```python
from build123d import *
from build123d.topology import SkipClean

# Parameters (mm, degrees)
CROQUIS2_R              = 11.9
SALIENTE_EXTRUIR1_DEPTH = 30
CROQUIS3_R              = 3
SALIENTE_EXTRUIR2_DEPTH = 1.5
CROQUIS4_R              = 1
CORTAR_EXTRUIR1_DEPTH   = 36.713722853
CROQUIS5_R              = 1.2
CORTAR_EXTRUIR2_DEPTH   = 5
CROQUIS7_R              = 4.5
SALIENTE_EXTRUIR3_DEPTH = 1.7
CORTAR_EXTRUIR3_REACH   = 39.222
CROQUIS8_R              = 1
SALIENTE_EXTRUIR4_DEPTH = 5
CORTAR_EXTRUIR4_REACH   = 41.632
CROQUIS10_R             = 0.5
CORTAR_EXTRUIR5_DEPTH   = 3
CORTAR_EXTRUIR7_DEPTH   = 2
SALIENTE_EXTRUIR5_START = 1
SALIENTE_EXTRUIR5_DEPTH = 1
CROQUIS16_R             = 1
SALIENTE_EXTRUIR8_DEPTH = 0.4
CROQUIS17_R             = 1
SALIENTE_EXTRUIR9_DEPTH = 45
REDONDEO4_R             = 0.2


with BuildPart() as part:
    # Croquis2 → Saliente-Extruir1 (new body)
    with BuildSketch(Plane.XY):
        Circle(CROQUIS2_R)
    extrude(amount=SALIENTE_EXTRUIR1_DEPTH)

    # Croquis3 → Saliente-Extruir2 (add)
    with BuildSketch(Plane.XY.offset(30)):
        Circle(CROQUIS3_R)
    extrude(amount=SALIENTE_EXTRUIR2_DEPTH)

    # Croquis4 → Cortar-Extruir1 (cut, through all)
    with BuildSketch(Plane.XY.offset(31.5)):
        Circle(CROQUIS4_R)
    extrude(amount=-CORTAR_EXTRUIR1_DEPTH, mode=Mode.SUBTRACT)

    # Croquis5 → Cortar-Extruir2 (cut)
    with BuildSketch(Plane.XY.offset(30)):
        with Locations((7, 0)):
            Circle(CROQUIS5_R)
        with Locations((-7, 0)):
            Circle(CROQUIS5_R)
    extrude(amount=-CORTAR_EXTRUIR2_DEPTH, mode=Mode.SUBTRACT)

    # Croquis7 → Saliente-Extruir3 (add)
    with BuildSketch(Plane(origin=(0, 0, 0), x_dir=(-1, 0, 0), z_dir=(0, 0, -1))):
        with Locations(Location((0, 0, 0), (0, 0, 180))):
            Circle(CROQUIS7_R)
    extrude(amount=SALIENTE_EXTRUIR3_DEPTH)

    # Croquis8 → Cortar-Extruir3 (cut, up to next)
    with BuildSketch(Plane(origin=(0, 0, -1.7), x_dir=(-1, 0, 0), z_dir=(0, 0, -1)), mode=Mode.PRIVATE) as cortar_extruir3_sk1:
        with Locations(Location((0, 0, 0), (0, 0, 180))):
            Circle(CROQUIS8_R)
    cortar_extruir3_tool1 = extrude(cortar_extruir3_sk1.sketch, amount=-CORTAR_EXTRUIR3_REACH, mode=Mode.PRIVATE) & part.part
    add(cortar_extruir3_tool1.solids().sort_by_distance((0, 0, -1.7))[0], mode=Mode.SUBTRACT)

    # Croquis9 → Saliente-Extruir4 (add)
    with BuildSketch(Plane(origin=(0, 0, 0), x_dir=(-1, 0, 0), z_dir=(0, 0, -1))):
        Polygon((-9, 0), (-9, 1.5), (-8.4, 1.5), (-8.4, -1.5), (-9, -1.5), align=None)
        Polygon((9, 0), (9, 1.5), (8.4, 1.5), (8.4, -1.5), (9, -1.5), align=None)
    extrude(amount=SALIENTE_EXTRUIR4_DEPTH)

    # Cortar-Extruir4: up to this face of the body (flat: up to its plane)
    cortar_extruir4_end = Plane(part.part.faces().sort_by_distance((9, 0, -2.5))[0])
    # Croquis10 → Cortar-Extruir4 (cut, up to the picked face)
    with BuildSketch(Plane.ZY.offset(9), mode=Mode.PRIVATE) as cortar_extruir4_sk1:
        with BuildLine():
            Line((-5, -1.5), (-3.5, -1.5))
            ThreePointArc((-3.5, -1.5), (-4.560660172, -1.060660172), (-5, 0))
            Line((-5, 0), (-5, -1.5))
        make_face()
    cortar_extruir4_tool1 = split(extrude(cortar_extruir4_sk1.sketch, amount=-CORTAR_EXTRUIR4_REACH, mode=Mode.PRIVATE), bisect_by=cortar_extruir4_end, keep=Keep.BOTH, mode=Mode.PRIVATE)
    # Croquis10 → Cortar-Extruir4 (cut, up to the picked face)
    with BuildSketch(Plane.ZY.offset(9), mode=Mode.PRIVATE) as cortar_extruir4_sk2:
        with BuildLine():
            Line((-5, 1.5), (-5, 0))
            ThreePointArc((-5, 0), (-4.560660172, 1.060660172), (-3.5, 1.5))
            Line((-3.5, 1.5), (-5, 1.5))
        make_face()
    cortar_extruir4_tool2 = split(extrude(cortar_extruir4_sk2.sketch, amount=-CORTAR_EXTRUIR4_REACH, mode=Mode.PRIVATE), bisect_by=cortar_extruir4_end, keep=Keep.BOTH, mode=Mode.PRIVATE)
    # Croquis10 → Cortar-Extruir4 (cut, up to the picked face)
    with BuildSketch(Plane.ZY.offset(9), mode=Mode.PRIVATE) as cortar_extruir4_sk3:
        with Locations((-3.5, 0)):
            Circle(CROQUIS10_R)
    cortar_extruir4_tool3 = split(extrude(cortar_extruir4_sk3.sketch, amount=-CORTAR_EXTRUIR4_REACH, mode=Mode.PRIVATE), bisect_by=cortar_extruir4_end, keep=Keep.BOTH, mode=Mode.PRIVATE)
    add(cortar_extruir4_tool1.solids().sort_by(Axis((-9, -1.164948, -4.664948), (1, 0, 0)))[0], mode=Mode.SUBTRACT)
    add(cortar_extruir4_tool2.solids().sort_by(Axis((-9, 1.164948, -4.664948), (1, 0, 0)))[0], mode=Mode.SUBTRACT)
    add(cortar_extruir4_tool3.solids().sort_by(Axis((-9, 0, -3.5), (1, 0, 0)))[0], mode=Mode.SUBTRACT)

    # Croquis11 → Cortar-Extruir5 (cut)
    with BuildSketch(Plane(origin=(0, 0, 0), x_dir=(-1, 0, 0), z_dir=(0, 0, -1))):
        with BuildLine():
            Line((-1.5, -10), (-1.5, -12.544656971))
            Line((-1.5, -12.544656971), (1.5, -12.544656971))
            Line((1.5, -12.544656971), (1.5, -10))
            ThreePointArc((1.5, -10), (0, -8.5), (-1.5, -10))
        make_face()
        with BuildLine():
            Line((-1.5, 10), (-1.5, 12.84563131))
            Line((-1.5, 12.84563131), (1.5, 12.84563131))
            Line((1.5, 12.84563131), (1.5, 10))
            ThreePointArc((1.5, 10), (0, 8.5), (-1.5, 10))
        make_face()
    extrude(amount=-CORTAR_EXTRUIR5_DEPTH, mode=Mode.SUBTRACT)

    # Croquis12 → Cortar-Extruir7 (cut)
    with SkipClean():  # the faces are left unmerged after this step: merging them gives an invalid solid
        with BuildSketch(Plane(origin=(0, 0, 0), x_dir=(-1, 0, 0), z_dir=(0, 0, -1))):
            with BuildLine():
                Line((-2, 4.031128874), (-2, 7.745966692))
                ThreePointArc((-2, 7.745966692), (-5.835121404, 5.472783405), (-7.858116823, 1.5))
                Line((-7.858116823, 1.5), (-8.4, 1.5))
                Line((-8.4, 1.5), (-8.4, -1.5))
                Line((-8.4, -1.5), (-7.858116823, -1.5))
                ThreePointArc((-7.858116823, -1.5), (-5.835121404, -5.472783405), (-2, -7.745966692))
                Line((-2, -7.745966692), (-2, -4.031128874))
                ThreePointArc((-2, -4.031128874), (-4.5, 0), (-2, 4.031128874))
            make_face()
            with BuildLine():
                Line((2, -4.031128874), (2, -7.745966692))
                ThreePointArc((2, -7.745966692), (5.835121404, -5.472783405), (7.858116823, -1.5))
                Line((7.858116823, -1.5), (8.4, -1.5))
                Line((8.4, -1.5), (8.4, 1.5))
                Line((8.4, 1.5), (7.858116823, 1.5))
                ThreePointArc((7.858116823, 1.5), (5.835121404, 5.472783405), (2, 7.745966692))
                Line((2, 7.745966692), (2, 4.031128874))
                ThreePointArc((2, 4.031128874), (4.5, 0), (2, -4.031128874))
            make_face()
            with BuildLine():
                Line((-9, -1.5), (-9, 1.5))
                Line((-9, 1.5), (-11.805083651, 1.5))
                ThreePointArc((-11.805083651, 1.5), (-11.9, 0), (-11.805083651, -1.5))
                Line((-11.805083651, -1.5), (-9, -1.5))
            make_face()
            with BuildLine():
                Line((9, 1.5), (9, -1.5))
                Line((9, -1.5), (11.805083651, -1.5))
                ThreePointArc((11.805083651, -1.5), (11.9, 0), (11.805083651, 1.5))
                Line((11.805083651, 1.5), (9, 1.5))
            make_face()
        extrude(amount=-CORTAR_EXTRUIR7_DEPTH, mode=Mode.SUBTRACT)

    # Croquis13 → Saliente-Extruir5 (add)
    with SkipClean():  # the faces are left unmerged after this step: merging them gives an invalid solid
        with BuildSketch(Plane(origin=(0, 0, 2), x_dir=(-1, 0, 0), z_dir=(0, 0, -1)).offset(SALIENTE_EXTRUIR5_START)):
            with BuildLine():
                Line((2, 4.582575695), (2, 4.031128874))
                ThreePointArc((2, 4.031128874), (4.5, 0), (2, -4.031128874))
                Line((2, -4.031128874), (2, -4.582575695))
                ThreePointArc((2, -4.582575695), (5, 0), (2, 4.582575695))
            make_face()
            with BuildLine():
                Line((-2, -4.582575695), (-2, -4.031128874))
                ThreePointArc((-2, -4.031128874), (-4.5, 0), (-2, 4.031128874))
                Line((-2, 4.031128874), (-2, 4.582575695))
                ThreePointArc((-2, 4.582575695), (-5, 0), (-2, -4.582575695))
            make_face()
        extrude(amount=-SALIENTE_EXTRUIR5_DEPTH)



with BuildPart() as body_2:
    # Croquis16 → Saliente-Extruir8 (new body)
    with BuildSketch(Plane(origin=(0, 0, -1.7), x_dir=(-1, 0, 0), z_dir=(0, 0, -1))):
        with Locations(Location((0, 0, 0), (0, 0, 180))):
            Circle(CROQUIS16_R)
    extrude(amount=SALIENTE_EXTRUIR8_DEPTH)


with BuildPart() as part_1:
    with SkipClean():  # the faces are left unmerged after this step: merging them gives an invalid solid
        add(part.part)

        add(body_2.part)  # Saliente-Extruir9 merges body 2
        # Croquis17 → Saliente-Extruir9 (add)
        with BuildSketch(Plane(origin=(0, 0, -2.1), x_dir=(-1, 0, 0), z_dir=(0, 0, -1))):
            Circle(CROQUIS17_R)
        extrude(amount=-SALIENTE_EXTRUIR9_DEPTH)

    # Redondeo4
    redondeo4_edges = [part_1.edges().sort_by_distance(p)[0] for p in [
        (1, 0, 42.9),
        (0, -1, -2.1),
    ]]
    fillet(redondeo4_edges, radius=REDONDEO4_R)


solid = part_1.part
```
Source: CAD feature listing. Evaluate the final solid. Frame: model axes, mm. A direction names the side the tool comes from. Give positions to 0.01 mm unless a question says otherwise; leave off trailing zeros. Loops run counter-clockwise (first coordinate to the right, second up) from the corner with the lowest first, then second, coordinate; pieces in that order, holes last. Notation, with made-up numbers: (-6, -38) -> (-2, -38) arc R16 ccw to (-2, -32) -> close; hole circle Ø9 at (42.5, 52). An arc over 180 degrees is marked (long way). Put each result on its own line as item: value. Start each with the question number.
1) Cut plane A-A (x = 10.5). Return loops of the section in (y, z).
2) Cut plane C-C (z = 32.5). Return loops of the section in (x, y), then the cut area to 3 significant figures.
3) Material intervals for probe 1 along Y at (x, z) = (-8.8, -3.5); probe 2 along Z at (x, y) = (-8.5, -2.5); probe 3 along X at (y, z) = (-0.5, 24.5), sorted ascending.
4) Cut plane D-D (x = 3.5). Return loops of the section in (y, z), then the cut area to 3 significant figures.
5) Draft query along Y for faces 4 (the face through (0, -8.5, 1.5)), 5 (the face through (5.8, 0.05, 27.54)), 6 (the face through (-3, 0, 31)). Return one class per face: released by +Y, released by -Y, zero draft, split by the parting line, or undercut.
6) Cut plane B-B (y = -6.25). Return loops of the section in (x, z).
7) Contact query for flat-ended pins moving along their axis: P1, Ø1.6, axis at x = 10.5, z = 1, coming from the -Y side; P2, Ø0.6, axis at x = 11, z = 0.5, coming from the +Y side; P3, Ø3, axis at x = -2, y = 5.5, coming from the +Z side; P4, Ø1, axis at x = -2, z = 36, coming from the +Y side. Output: stop coordinate, or through.
8) Reachability of faces 1 (the face through (-5.2, 0.1, 2)), 2 (the face through (-1.5, 11, 1)), 3 (the face through (-10, -1.5, 1)) from +Z, -Z, +X, -X, +Y, -Y: full face, straight path, thin tool, end or side. Return the list, or none.
Results are:
1. outline: (-5.6, 0) -> (-1.5, 0) -> (-1.5, 2) -> (1.5, 2) -> (1.5, 0) -> (5.6, 0) -> (5.6, 30) -> (-5.6, 30) -> close
2. outline: circle Ø2 at (0, 0)
2. area: 3.14 mm2
3. probe 1: y = -1.5 to -0.5, 0.5 to 1.5
3. probe 2: z = 0 to 30
3. probe 3: x = -11.89 to 11.89
4. outline: (-11.37, 0) -> (-7.19, 0) -> (-7.19, 2) -> (-3.57, 2) -> (-3.57, 1) -> (-2.83, 1) -> (-2.83, -1.7) -> (2.83, -1.7) -> (2.83, 1) -> (3.57, 1) -> (3.57, 2) -> (7.19, 2) -> (7.19, 0) -> (11.37, 0) -> (11.37, 30) -> (-11.37, 30) -> close
4. area: 676 mm2
5. face 4: released by -Y
5. face 5: undercut
5. face 6: split by the parting line
6. outline: (-10.13, 0) -> (-4.99, 0) -> (-4.99, 2) -> (-2, 2) -> (-2, 0) -> (2, 0) -> (2, 2) -> (4.99, 2) -> (4.99, 0) -> (10.13, 0) -> (10.13, 30) -> (-10.13, 30) -> close
7. P1: stops at y = -6.89
7. P2: stops at y = 5.21
7. P3: stops at z = 30
7. P4: passes through
8. face 1: -Z
8. face 2: -Z, +Y
8. face 3: -Z, -X
